The figure shows three views and two pictorial views of one solid part (mm, origin at its lowest corner). Answer the questions. Coordinates: 2 decimals unless noted, no trailing zeros. Order: outer loops, then holes, each group sorted by start corner. A loop starts at its lowest first (then second) coordinate and runs counter-clockwise, first axis right, second up.
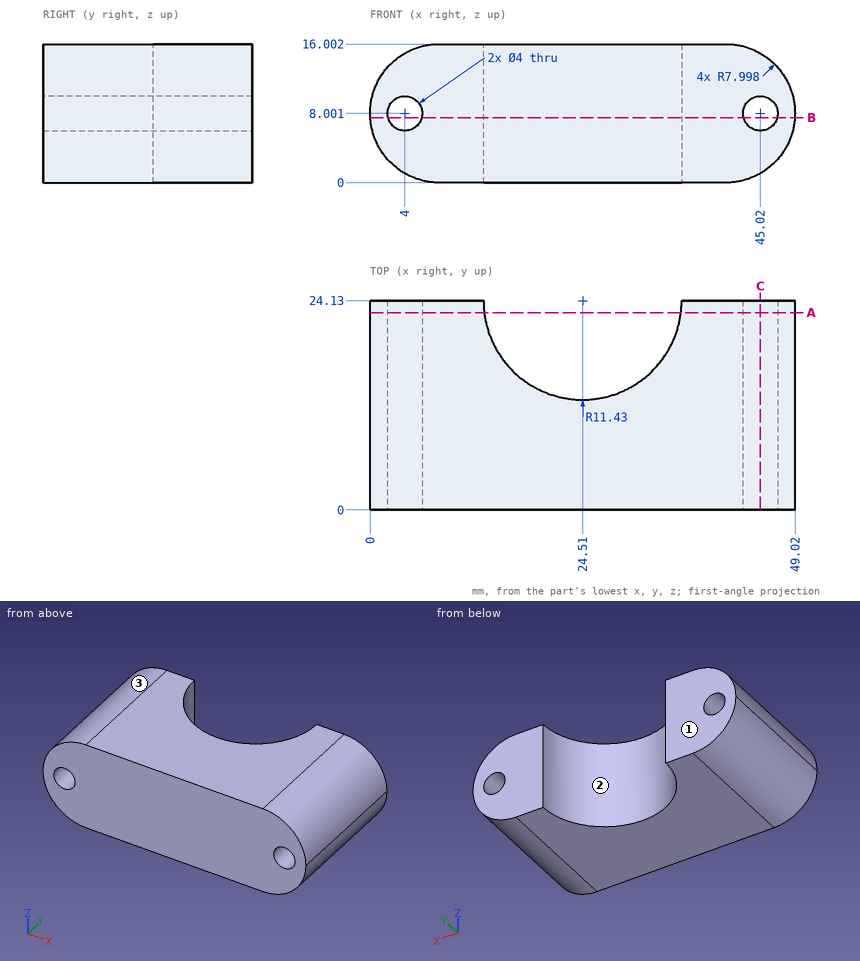
Q1. The part is cut by section C-C, the plane x = 45.02. Determine the outline of the cut face in (y, z).
Q2. Straight lines are drawn through the part: L1, parallel to X at y = 10.25, z = 8.75 (1 decimal); L2, parallel to Z at x = 3.5, y = 4.25 (1 decimal); L3, parallel to Z at x = 45.02, y = 12. For each, find the intervals that lie inside material, in ascending order.
Q3. Each of these flat-tipped pins is pushed along its axis until it touches: P1, Ø1.5, axis at y = 15.5, z = 10.5, coming from the +X side; P2, Ø3, axis at y = 5.5, z = 4, coming from the +X side; P3, Ø6, axis at x = 21.5, z = 14.5, coming from the +Y side. Where does it stop, or does it pass through?
Q4. Determine the mould class of the marked faces 1, 2 and 3 for opening direction X: +X half, -X half, draft (parallel to the pull), parting line (faces both ways), or undercut.
Q5. The part is cut by section A-A, the plane y = 22.75. State how many separate pieces and enclosed holes the cut face has, then the cut area to 3 significant figures.
Q6. The part is cut by section B-B, the plane z = 7.5. Determine the outline of the cut face in (x, y) (1 decimal), then the cut area to 3 significant figures.
Computed values:
1. outline: (0, 1.07) - (24.13, 1.07) - (24.13, 6) - (0, 6) - close; (0, 10) - (24.13, 10) - (24.13, 14.93) - (0, 14.93) - close
2. L1: x = 0 to 2.1, 5.9 to 43.2, 46.9 to 49
2. L2: z = 1.4 to 6.1, 9.9 to 14.6
2. L3: z = 1.07 to 6, 10 to 14.93
3. P1: stops at x = 48.83
3. P2: stops at x = 48.62
3. P3: stops at y = 14.41
4. face 1: draft
4. face 2: undercut
4. face 3: -X half
5. separate pieces: 2
5. enclosed holes: 2
5. area: 341 mm2
6. outline: (0, 0) - (2.1, 0) - (2.1, 24.1) - (0, 24.1) - close; (5.9, 0) - (43.1, 0) - (43.1, 24.1) - (35.9, 24.1) arc R11.4 cw to (13.1, 24.1) - (5.9, 24.1) - close; (47, 0) - (49, 0) - (49, 24.1) - (47, 24.1) - close
6. area: 790 mm2
